Autodesk Inventor part; units mm, degrees
ref_plane "YZ Plane" through (0, 0, 0) normal (1, 0, 0) x (0, 1, 0)
ref_plane "XZ Plane" through (0, 0, 0) normal (0, 1, 0) x (-1, 0, 0)
ref_plane "XY Plane" through (0, 0, 0) normal (0, 0, 1) x (1, 0, 0)
sketch "Sketch5" plane through (0, 0, 0) normal (0, 0, 1) x (1, 0, 0)
  circle A0 centre (0, 0) radius 14.35
  circle A1 centre (0, 0) radius 17.15
  line L0 (0, 0) -> (20, 0)
  line L1 (20, 0) -> (20, 20)
  line L2 (20, 20) -> (0, 20)
  line L3 (0, 20) -> (0, 0)
  line L4 (20, 20) -> (-20, 20)
  line L5 (-20, 20) -> (-20, -20)
  line L6 (-20, -20) -> (20, -20)
  line L7 (20, -20) -> (20, 20)
  dimension "d36" = 28.7
  dimension "d37" = 34.3
  dimension "d54" = 20
  dimension "d55" = 20
  dimension "d56" = 40
  dimension "d57" = 40
extrude "Extrusion10" add sketch "Sketch5" along normal blind 10
sketch "Sketch8" plane through (0, 0, 0) normal (0, 0, -1) x (-1, 0, 0)
  circle A0 centre (0, 0) radius 14.35
  circle A1 centre (0, 0) radius 17.15
  circle A2 centre (0, 0) radius 14.35
  circle A3 centre (0, 0) radius 17.15
  dimension "d60" = 28.7
  dimension "d61" = 34.3
  dimension "d62" = 28.7
  dimension "d63" = 34.3
extrude "Extrusion11" cut sketch "Sketch8" against normal blind 5
properties part number "Clip_MarkerHolderV1"
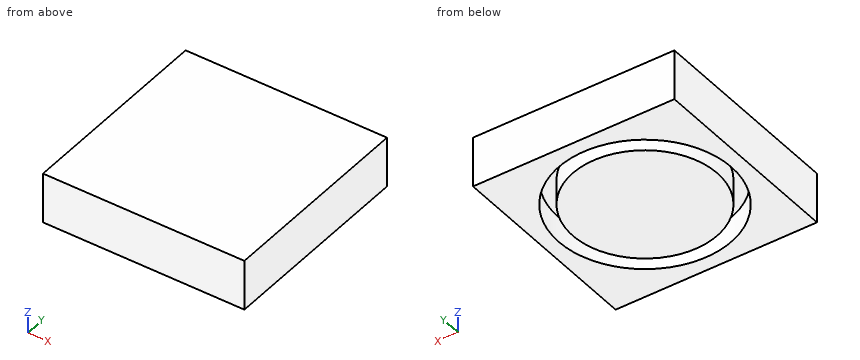
The listing builds one solid part. Answer for the finished solid, in the listing's coordinates (mm). Give positions to 0.01 mm unless a question says otherwise; leave off trailing zeros. Write each loop counter-clockwise with the first axis right and the second up, starting at its lowest first coordinate (ties: lowest second). Pieces come first, ordered by that corner, then holes. Notation, with made-up numbers: (3.25, -34.5) - (44.25, -34.5) arc R11 cw to (44.25, -21.5) - close; hole circle Ø10 at (63, -4). An arc over 180 degrees is marked (long way). One line per question, with ' | ' between items. Start each with the question number.
1. Straight lines are drawn through the part: line 1 (Y direction, x = 0, z = 3.8); line 2 (Y direction, x = 12, z = 4.5); line 3 (Z direction, x = -15.5, y = 6.5). For each, find the intervals that lie inside material, in ascending order.
2. Section B-B, the plane x = 0 is taken. Determine the outline of the cut face in (y, z), then the cut area to 3 significant figures.
3. Section D-D, the plane y = 15.5 is taken. Determine the outline of the cut face in (x, z).
4. Section A-A, the plane z = 1.75 is taken. Determine the outline of the cut face in (x, y).
Result:
1) line 1: y = -20 to -17.15, -14.35 to 14.35, 17.15 to 20 | line 2: y = -20 to -12.25, -7.87 to 7.87, 12.25 to 20 | line 3: z = 5 to 10
2) outline: (-20, 0) - (-17.15, 0) - (-17.15, 5) - (-14.35, 5) - (-14.35, 0) - (14.35, 0) - (14.35, 5) - (17.15, 5) - (17.15, 0) - (20, 0) - (20, 10) - (-20, 10) - close | area: 372 mm2
3) outline: (-20, 0) - (-7.34, 0) - (-7.34, 5) - (7.34, 5) - (7.34, 0) - (20, 0) - (20, 10) - (-20, 10) - close
4) outline: (-20, -20) - (20, -20) - (20, 20) - (-20, 20) - close; circle Ø28.7 at (0, 0); hole circle Ø34.3 at (0, 0)
